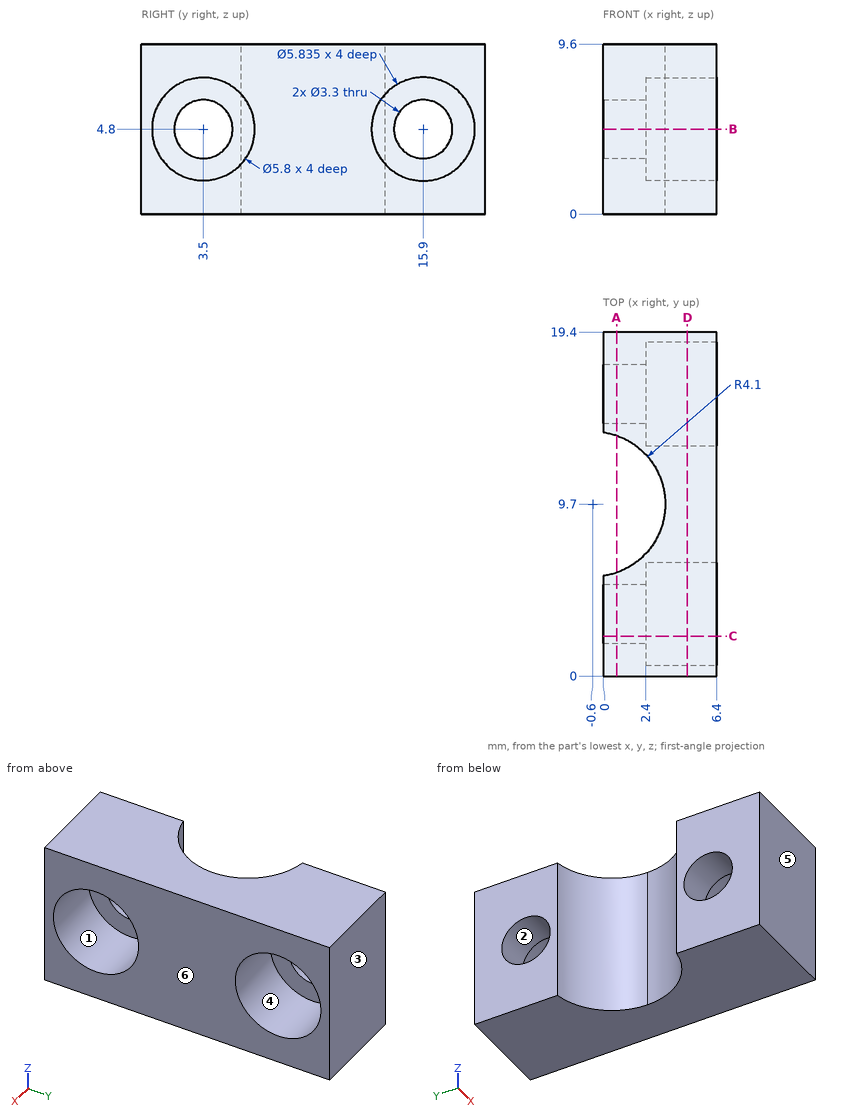
Study the drawing (mm; zero at the part's minimum x, y, z) and answer. A direction names the side the tool comes from. Round coordinates to 2 decimals unless told otherwise and drop trailing zeros. Loops run counter-clockwise (first coordinate to the right, second up) from the corner with the lowest first, then second, coordinate; pieces in that order, holes last.
Q1. For a pull along Y with two mould halves and no side action, classify the marked faces 3, 4, 5 and 6 as released by +Y, released by -Y, zero draft, split by the parting line, or undercut.
Q2. Section A-A, the plane x = 0.75 is taken. Determine the outline of the cut face in (y, z).
Q3. Section D-D, the plane x = 4.75 is taken. Determine the outline of the cut face in (y, z) (1 decimal).
Q4. Section B-B, the plane z = 4.8 is taken. Determine the outline of the cut face in (x, y).
Q5. Section C-C, the plane y = 2.25 is taken. Determine the outline of the cut face in (x, z).
Q6. Given pin 1 Ø1.5 at (x, z) = (0.5, 7.5) entering from -Y; pin 2 Ø1.8 at (y, z) = (17, 6) entering from +X; pin 3 Ø1.5 at (y, z) = (12.5, 7) entering from -X; pin 4 Ø5 at (y, z) = (9, 3) entering from -X (1 decimal), each flat-ended and moving along its own axis, determine where each tip first touches the part or whether it passes through.
Q7. Which of the six approach directions +Z, -Z, +X, -X, +Y, -Y give full straight-line access (tool end or side, diameter ignored) to the marked faces 1 and 2?
Q8. Find the intervals of material crossed by line 1 (Y direction, x = 4.75, z = 6.5); line 2 (Z direction, x = 3.45, y = 3.5); line 3 (Y direction, x = 6.25, z = 3.5), in increasing order.
Completed:
1. face 3: released by +Y
1. face 4: undercut
1. face 5: released by -Y
1. face 6: zero draft
2. outline: (0, 0) - (5.83, 0) - (5.83, 9.6) - (0, 9.6) - close; (13.57, 0) - (19.4, 0) - (19.4, 9.6) - (13.57, 9.6) - close; hole circle Ø3.3 at (3.5, 4.8); hole circle Ø3.3 at (15.9, 4.8)
3. outline: (0, 0) - (19.4, 0) - (19.4, 9.6) - (0, 9.6) - close; hole circle Ø5.8 at (3.5, 4.8); hole circle Ø5.8 at (15.9, 4.8)
4. outline: (0, 0) - (6.4, 0) - (6.4, 0.6) - (2.4, 0.6) - (2.4, 1.85) - (0, 1.85) - close; (0, 5.15) - (2.4, 5.15) - (2.4, 6.4) - (6.4, 6.4) - (6.4, 12.98) - (2.4, 12.98) - (2.4, 14.25) - (0, 14.25) - (0, 13.76) arc R4.1 cw to (3.5, 9.7) arc R4.1 cw to (0, 5.64) - close; (0, 17.55) - (2.4, 17.55) - (2.4, 18.82) - (6.4, 18.82) - (6.4, 19.4) - (0, 19.4) - close
5. outline: (0, 0) - (6.4, 0) - (6.4, 2.18) - (2.4, 2.18) - (2.4, 3.72) - (0, 3.72) - close; (0, 5.88) - (2.4, 5.88) - (2.4, 7.42) - (6.4, 7.42) - (6.4, 9.6) - (0, 9.6) - close
6. pin 1: stops at y = 0
6. pin 2: stops at x = 2.4
6. pin 3: stops at x = 1.45
6. pin 4: stops at x = 2
7. face 1: +X
7. face 2: +X, -X
8. line 1: y = 0 to 1.15, 5.85 to 13.53, 18.27 to 19.4
8. line 2: z = 0 to 1.9, 7.7 to 9.6
8. line 3: y = 0 to 0.91, 6.09 to 13.29, 18.51 to 19.4
